The drawing under review shows one solid part. Ordinate dimensions are in mm from its lowest x, y, z. A direction names the side the tool comes from. Coordinates: 2 decimals unless noted, no trailing zeros. Write each loop counter-clockwise with the first axis right and the second up, starting at its lowest first coordinate (ties: lowest second). Pieces come first, ordered by that corner, then holes. Notation, with made-up numbers: (48, 47.25) -> (66, 47.25) arc R18 cw to (66, 56.25) -> close; hole circle Ø2 at (-7, -13). An arc over 180 degrees is marked (long way). One line per question, with ' | ' between items. Start each with the question number.
Q1. Add section B-B on z = 9.35. State the section outline as (x, y) points.
Q2. Add section A-A on y = 0.55. State the section outline as (x, z) points.
Q3. For the marked faces 5 and 6, list the 3-axis set-ups (+Z, -Z, +X, -X, +Y, -Y) from which the entire face can be reached by the end or side of a thin tool; tool diameter is ignored.
Q4. Add section D-D on y = 3.8. State the section outline as (x, z) points.
Q5. For P1, Ø1.8, axis at x = 3.5, y = 1.5, coming from the -Z side; P2, Ø1.5, axis at x = 2, z = 13, coming from the -Y side, all flat-tipped, find the tip position at first contact; note any pin that passes through.
Q6. Wall thickness on probe 1 along Z at (x, y) = (5, 3.95); probe 2 along Z at (x, y) = (1.25, 1.8); probe 3 along Y at (x, z) = (9.75, 10): over which ranges is each line inside the solid? List them lowest first.
Q7. Add section C-C on x = 5. State the section outline as (y, z) points.
Q8. Draft analysis for pull direction Z (two halves, no side actions). For the marked faces 1, 2, 3 and 4, state which applies: pulls with the +Z half, pulls with the -Z half, needs draft (parallel to the pull), parting line crosses it, or undercut.
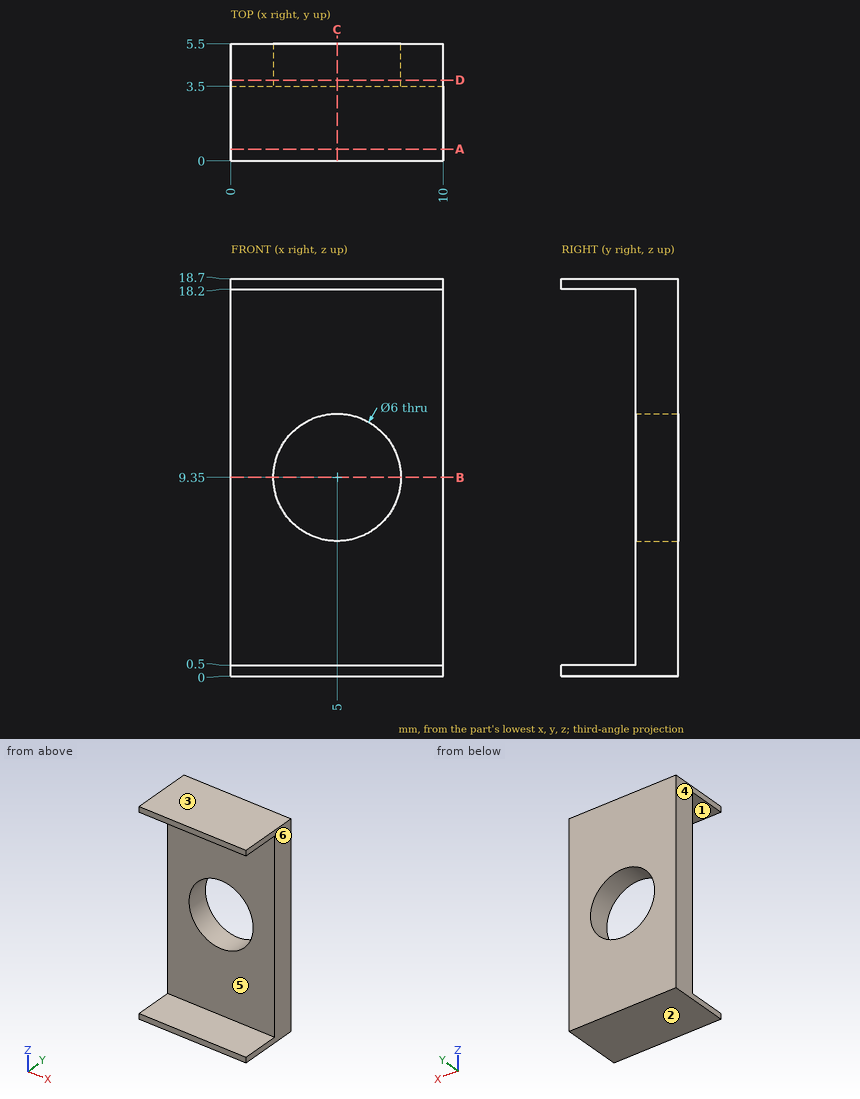
Output values:
1) outline: (0, 3.5) -> (2, 3.5) -> (2, 5.5) -> (0, 5.5) -> close; (8, 3.5) -> (10, 3.5) -> (10, 5.5) -> (8, 5.5) -> close
2) outline: (0, 0) -> (10, 0) -> (10, 0.5) -> (0, 0.5) -> close; (0, 18.2) -> (10, 18.2) -> (10, 18.7) -> (0, 18.7) -> close
3) face 5: +X, -X, -Y | face 6: +Z, -Z, +X, +Y, -Y
4) outline: (0, 0) -> (10, 0) -> (10, 18.7) -> (0, 18.7) -> close; hole circle Ø6 at (5, 9.35)
5) P1: stops at z = 0 | P2: stops at y = 3.5
6) probe 1: z = 0 to 6.35, 12.35 to 18.7 | probe 2: z = 0 to 0.5, 18.2 to 18.7 | probe 3: y = 3.5 to 5.5
7) outline: (0, 0) -> (5.5, 0) -> (5.5, 6.35) -> (3.5, 6.35) -> (3.5, 0.5) -> (0, 0.5) -> close; (0, 18.2) -> (3.5, 18.2) -> (3.5, 12.35) -> (5.5, 12.35) -> (5.5, 18.7) -> (0, 18.7) -> close
8) face 1: undercut | face 2: pulls with the -Z half | face 3: pulls with the +Z half | face 4: needs draft
